Source: CAD feature listing. Evaluate the final solid. Frame: model axes, mm. A direction names the side the tool comes from. Round coordinates to 2 decimals unless told otherwise and drop trailing zeros. Order: outer loops, then holes, each group sorted by start corner. A loop starts at its lowest first (then second) coordinate and runs counter-clockwise, first axis right, second up. Notation, with made-up numbers: (29, -20) - (37, -20) arc R25 ccw to (37, 11) - close; hole circle Ø8 at (-17.75, -36). An arc over 180 degrees is marked (long way). Use one line per item in the form item = value. Start each with the question number.
Q1. Cut plane D-D, the plane x = 13. Return the cut outline in (y, z), and give its area (3 significant figures).
Q2. Pin query (flat end, axial travel): pin 1 Ø11 at (x, z) = (77, 4) entering from -Y; pin 2 Ø3.5 at (x, y) = (61.5, 52.5) entering from +Z; pin 3 Ø1 at (y, z) = (2.5, 1) entering from -X. Return the tip coordinate at first contact, or that it passes through.
Q3. Cut plane A-A, the plane z = 9.75. Return the cut outline in (x, y), and give its area (3 significant figures).
Q4. Set-up query: faces 4 (the cylindrical face through (64.457, 4.431, -0.246)), 5 (the flat face through (32, 5, 2)), 6 (the flat face through (32, -1.292, 1)), 7 (the flat face through (47.654, 12, 2)), 8 (the flat face through (32, 10.833, 1)). Return all of +Z, -Z, +X, -X, +Y, -Y with unobstructed straight access to the full face (end or side cutting, diameter ignored); none if empty.
Q5. Draft query along Y for faces 1 (the flat face through (53, 0, 3)), 2 (the cylindrical face through (84.14, 55.1, -2.03)), 3 (the cylindrical face through (2.828, 6.526, -3.746)). Return one class per face: released by +Y, released by -Y, zero draft, split by the parting line, or undercut.
Q6. Cut plane B-B, the plane z = -2.25. Return the cut outline in (x, y) (3 decimals), and give its area (3 significant figures).
Q7. Cut plane C-C, the plane y = 27.5. Return the cut outline in (x, z), and give its area (3 significant figures).
Q8. Ray query, line 1 (Y direction, x = 3.5, z = -1.75) (3 decimals); line 2 (X direction, y = 52.5, z = -3.75); line 3 (Y direction, x = 61.5, z = -0.15). Return the intervals inside material, ascending. Write a range as [from, to].
from build123d import *

# Parameters (mm, degrees)
EXTRUDE_START       = -4
EXTRUDE_2_DEPTH     = 4
SKETCH_2_R          = 3.1
CUT_EXTRUDE_1_DEPTH = 0.5
SKETCH_3_R          = 1.375
CUT_EXTRUDE_2_DEPTH = 4
SKETCH_4_W          = 50.8
SKETCH_4_H          = 5.08
EXTRUDE_3_DEPTH     = 6
SKETCH_5_W          = 12.235874624
SKETCH_5_H          = 11.932505832
EXTRUDE_4_DEPTH     = 1
SKETCH_6_W          = 17.407120639
SKETCH_6_H          = 13.510004078
SKETCH_6_H_2        = 13.120292422
EXTRUDE_5_DEPTH     = 14
SKETCH_7_W          = 21.748003317
SKETCH_7_H          = 15.815488158
EXTRUDE_6_DEPTH     = 15
SKETCH_8_W          = 9.2021867
SKETCH_8_H          = 8.797694978
EXTRUDE_7_DEPTH     = 1
SKETCH_9_W          = 14.519457286
SKETCH_9_H          = 12.125029798
EXTRUDE_8_DEPTH     = 2
SKETCH_10_W         = 7
SKETCH_10_H         = 12.812960392
EXTRUDE_9_DEPTH     = 7
SKETCH_11_R         = 3
SKETCH_11_R_2       = 2
EXTRUDE_1_DEPTH     = 2
EXTRUDE_10_DEPTH    = 4
SKETCH_13_W         = 7.492652901
SKETCH_13_H         = 5.40798094
EXTRUDE_11_DEPTH    = 1
EXTRUDE_12_DEPTH    = 4
CUT_EXTRUDE_START   = -0.5
SKETCH_15_R         = 3.1
CUT_EXTRUDE_3_DEPTH = 0.5


# Read off the part's stored shape, not the designer's step: 凸台-拉伸2
with BuildPart() as part:
    # 凸台-拉伸2 outline → 凸台-拉伸2 (new body)
    with BuildSketch(Plane.XY.offset(EXTRUDE_START)):
        with BuildLine():
            ThreePointArc((3, 56), (0.878679656, 55.121320344), (0, 53))
            Line((0, 53), (0, 3))
            ThreePointArc((0, 3), (0.878679656, 0.878679656), (3, 0))
            Line((3, 0), (82, 0))
            ThreePointArc((82, 0), (84.121320344, 0.878679656), (85, 3))
            Line((85, 3), (85, 53))
            ThreePointArc((85, 53), (84.121320344, 55.121320344), (82, 56))
            Line((82, 56), (3, 56))
        make_face()
    extrude(amount=EXTRUDE_2_DEPTH)

    # 草图2 → 切除-拉伸1 (cut)
    with BuildSketch(Plane.XY):
        with Locations((3.5, 3.5)):
            Circle(SKETCH_2_R)
        with Locations((61.5, 3.5)):
            Circle(SKETCH_2_R)
        with Locations((3.5, 52.5)):
            Circle(SKETCH_2_R)
        with Locations((61.5, 52.5)):
            Circle(SKETCH_2_R)
    extrude(amount=-CUT_EXTRUDE_1_DEPTH, mode=Mode.SUBTRACT)

    # 草图3 → 切除-拉伸2 (cut)
    with BuildSketch(Plane.XY):
        with Locations((3.5, 52.5)):
            Circle(SKETCH_3_R)
        with Locations((61.5, 52.5)):
            Circle(SKETCH_3_R)
        with Locations((3.5, 3.5)):
            Circle(SKETCH_3_R)
        with Locations((61.5, 3.5)):
            Circle(SKETCH_3_R)
    extrude(amount=-CUT_EXTRUDE_2_DEPTH, mode=Mode.SUBTRACT)

    # 草图4 → 凸台-拉伸3 (add)
    with BuildSketch(Plane.XY):
        with Locations((32.682745254, 52.232035351)):
            Rectangle(SKETCH_4_W, SKETCH_4_H)
    extrude(amount=EXTRUDE_3_DEPTH)

    # 草图5 → 凸台-拉伸4 (add)
    with BuildSketch(Plane.XY):
        with Locations((29.806273598, 30.264010216)):
            Rectangle(SKETCH_5_W, SKETCH_5_H)
    extrude(amount=EXTRUDE_4_DEPTH)

    # 草图6 → 凸台-拉伸5 (add)
    with BuildSketch(Plane.XY):
        with Locations((78.345183612, 46.994971673)):
            Rectangle(SKETCH_6_W, SKETCH_6_H)
        with Locations((78.345183612, 28.873379664)):
            Rectangle(SKETCH_6_W, SKETCH_6_H_2)
    extrude(amount=EXTRUDE_5_DEPTH)

    # 草图7 → 凸台-拉伸6 (add)
    with BuildSketch(Plane.XY):
        with Locations((76.314084713, 10.301990913)):
            Rectangle(SKETCH_7_W, SKETCH_7_H)
    extrude(amount=EXTRUDE_6_DEPTH)

    # 草图8 → 凸台-拉伸7 (add)
    with BuildSketch(Plane.XY):
        with Locations((57.716202493, 34.157243051)):
            Rectangle(SKETCH_8_W, SKETCH_8_H)
    extrude(amount=EXTRUDE_7_DEPTH)

    # 草图9 → 凸台-拉伸8 (add)
    with BuildSketch(Plane.XY):
        with Locations((32.383118315, 4.770804671)):
            Rectangle(SKETCH_9_W, SKETCH_9_H)
    extrude(amount=EXTRUDE_8_DEPTH)

    # 草图10 → 凸台-拉伸9 (add)
    with BuildSketch(Plane.XY):
        with Locations((53.659033893, 6.406480196)):
            Rectangle(SKETCH_10_W, SKETCH_10_H)
    extrude(amount=EXTRUDE_9_DEPTH)

    # 草图11 → 拉伸-薄壁1 (add)
    with BuildSketch(Plane(origin=(0, 0, 0), x_dir=(-1, 0, 0), z_dir=(0, -1, 0))):
        with Locations((-53.5, -3.5)):
            Circle(SKETCH_11_R)
        with Locations((-53.5, -3.5)):
            Circle(SKETCH_11_R_2, mode=Mode.SUBTRACT)
    extrude(amount=EXTRUDE_1_DEPTH)

    # 草图12 → 凸台-拉伸10 (add)
    with BuildSketch(Plane.XY):
        Polygon((43.726404027, 3.853526794), (43.726404027, 0.513143902), (46.402655395, 0.513143902), (46.402655395, 3.853526794), (47.65405595, 5.104927349), (47.65405595, 18.391456575), (46.402655395, 19.64285713), (46.402655395, 22.77278121), (43.726404027, 22.77278121), (43.726404027, 19.64285713), (44.555447726, 19.64285713), (44.555447726, 3.853526794), align=None)
    extrude(amount=EXTRUDE_10_DEPTH)

    # 草图13 → 凸台-拉伸11 (add)
    with BuildSketch(Plane.XY):
        with Locations((10.870809128, 2.254112914)):
            Rectangle(SKETCH_13_W, SKETCH_13_H)
    extrude(amount=EXTRUDE_11_DEPTH)

    # 草图14 → 凸台-拉伸12 (add)
    with BuildSketch(Plane.XY):
        Polygon((2.981536039, 17.027603439), (5.803149545, 17.027603439), (5.803149545, 20.162023057), (4.903155557, 20.162023057), (4.903155557, 35.905554668), (5.803149545, 35.905554668), (5.803149545, 39.436558403), (2.981536039, 39.436558403), (2.981536039, 35.905554668), (1.735405071, 34.659423699), (1.735405071, 21.530793828), (2.981536039, 20.28466286), align=None)
    extrude(amount=EXTRUDE_12_DEPTH)

    # 草图15 → 切除-拉伸3 (cut)
    with BuildSketch(Plane(origin=(0, 0, -4), x_dir=(-1, 0, 0), z_dir=(0, 0, -1)).offset(CUT_EXTRUDE_START)):
        with Locations(Location((-61.5, 52.5, 0), (0, 0, 180))):
            Circle(SKETCH_15_R)
        with Locations(Location((-61.5, 3.5, 0), (0, 0, 180))):
            Circle(SKETCH_15_R)
        with Locations(Location((-3.5, 52.5, 0), (0, 0, 180))):
            Circle(SKETCH_15_R)
        with Locations(Location((-3.5, 3.5, 0), (0, 0, 180))):
            Circle(SKETCH_15_R)
    extrude(amount=CUT_EXTRUDE_3_DEPTH, mode=Mode.SUBTRACT)


solid = part.part
Completed:
q1.outline = (-0.45, 0) - (0, 0) - (0, -4) - (56, -4) - (56, 0) - (54.77, 0) - (54.77, 6) - (49.69, 6) - (49.69, 0) - (4.96, 0) - (4.96, 1) - (-0.45, 1) - close
q1.area = 260 mm2
q2.pin_1 = 0
q2.pin_2 = -0.5
q2.pin_3 = 7.12
q3.outline = (65.44, 2.39) - (87.19, 2.39) - (87.19, 18.21) - (65.44, 18.21) - close; (69.64, 22.31) - (87.05, 22.31) - (87.05, 35.43) - (69.64, 35.43) - close; (69.64, 40.24) - (87.05, 40.24) - (87.05, 53.75) - (69.64, 53.75) - close
q3.area = 808 mm2
q4.face_4 = +Z
q4.face_5 = +Z, -X, -Y
q4.face_6 = +Z, -Z, -X, -Y
q4.face_7 = +Z, -Y
q4.face_8 = +Z, -X
q5.face_1 = released by -Y
q5.face_2 = released by +Y
q5.face_3 = undercut
q6.outline = (0, 3) arc R3 ccw to (3, 0) - (82, 0) arc R3 ccw to (85, 3) - (85, 53) arc R3 ccw to (82, 56) - (3, 56) arc R3 ccw to (0, 53) - close; hole circle Ø2.75 at (3.5, 3.5); hole circle Ø2.75 at (3.5, 52.5); hole circle Ø2.75 at (61.5, 3.5); hole circle Ø2.75 at (61.5, 52.5)
q6.area = 4,730 mm2
q7.outline = (0, -4) - (85, -4) - (85, 0) - (87.05, 0) - (87.05, 14) - (69.64, 14) - (69.64, 0) - (35.92, 0) - (35.92, 1) - (23.69, 1) - (23.69, 0) - (4.9, 0) - (4.9, 4) - (1.74, 4) - (1.74, 0) - (0, 0) - close
q7.area = 609 mm2
q8.line_1 = [0, 2.125], [4.875, 51.125], [53.875, 56]
q8.line_2 = [0, 0.4], [6.6, 58.4], [64.6, 85]
q8.line_3 = [0, 0.4], [6.6, 49.4], [55.6, 56]
